Part print with two shaded views. Sizes in mm from the minimum x, y, z corner. Give positions to 0.01 mm unless a question says otherwise; leave off trailing zeros. Order: outer loops, then holes, each group sorted by start corner. A loop starts at its lowest first (then second) coordinate and runs counter-clockwise, first axis right, second up. Notation, with made-up numbers: M 41.5,-3.5 L 45.5,-3.5 A17 cw 45.5,13.5 Z; hole C 22.25,80.25 d2. An arc over 180 degrees is marked long. Return JSON: item names as keys, results as strings.
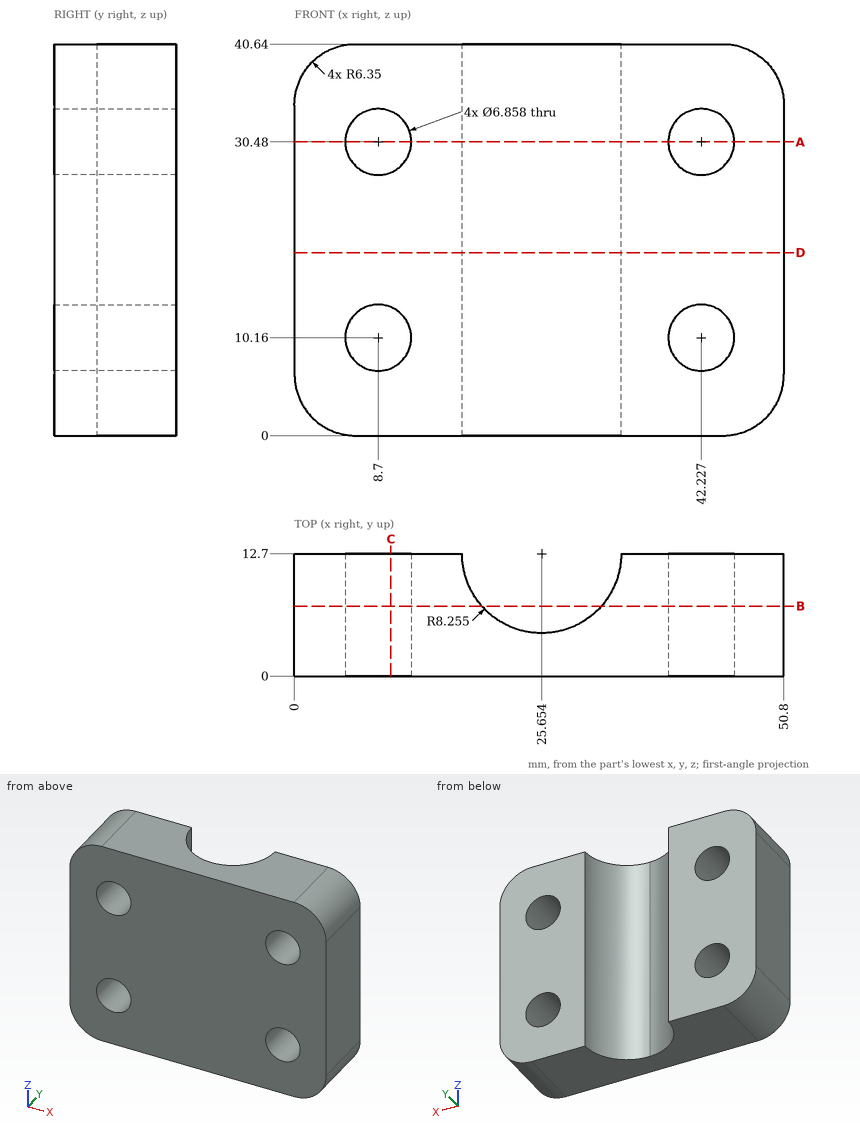
Q1. Pin check, flat tip, straight feed: pin 1 (9 mm diameter, centred on x = 42.23, z = 30.48, fed in from +Y). Stop position of the tip, or through.
Established:
{"pin 1": "stops at y = 12.7"}
Q2. Band-saw the part on A-A (z = 30.48). Give the cut face in (x, y) (1 decimal).
Established:
{"outline": "M 0,0 L 5.3,0 L 5.3,12.7 L 0,12.7 Z; M 12.1,0 L 38.8,0 L 38.8,12.7 L 33.9,12.7 A8.3 cw 17.4,12.7 L 12.1,12.7 Z; M 45.7,0 L 50.8,0 L 50.8,12.7 L 45.7,12.7 Z"}
Q3. Band-saw the part on D-D (z = 19). Give the cut face in (x, y) (1 decimal), then the cut area to 3 significant figures.
Established:
{"outline": "M 0,0 L 50.8,0 L 50.8,12.7 L 33.9,12.7 A8.3 cw 17.4,12.7 L 0,12.7 Z", "area": "538 mm²"}
Q4. Band-saw the part on B-B (y = 7.25). Give the number of separate pieces and of enclosed holes in the cut face, then the cut area to 3 significant figures.
Established:
{"separate pieces": "2", "enclosed holes": "4", "area": "1,380 mm²"}
Q5. Probe line 1 along X through (y, z) = (3.25, 30.48); line 2 along Z through (x, y) = (10.5, 3.75); line 3 along X through (y, z) = (9, 8) (1 decimal). List the from-to ranges inside material, lowest first.
Established:
{"line 1": "x = 0 to 5.27, 12.13 to 38.8, 45.66 to 50.8", "line 2": "z = 0 to 7.24, 13.08 to 27.56, 33.4 to 40.64", "line 3": "x = 0 to 6, 11.4 to 18.3, 33 to 39.6, 44.9 to 50.8"}
Q6. Band-saw the part on C-C (x = 10). Give the cut face in (y, z), then the cut area to 3 significant figures.
Established:
{"outline": "M 0,0 L 12.7,0 L 12.7,6.99 L 0,6.99 Z; M 0,13.33 L 12.7,13.33 L 12.7,27.31 L 0,27.31 Z; M 0,33.65 L 12.7,33.65 L 12.7,40.64 L 0,40.64 Z", "area": "355 mm²"}
